Verification items for this drawing (mm, ordinates from the low corner). Give positions to 0.01 mm unless a question says otherwise; leave off trailing zeros. Write each loop counter-clockwise with the first axis right and the second up, starting at its lowest first coordinate (ties: lowest second). Pieces come first, ordered by that corner, then holes. Notation, with made-up numbers: (-20.75, -9) -> (23.25, -9) arc R18 ccw to (23.25, 26) -> close; hole circle Ø4 at (-7, 67.25). An arc over 180 degrees is marked (long way). Write item = value, one per line.
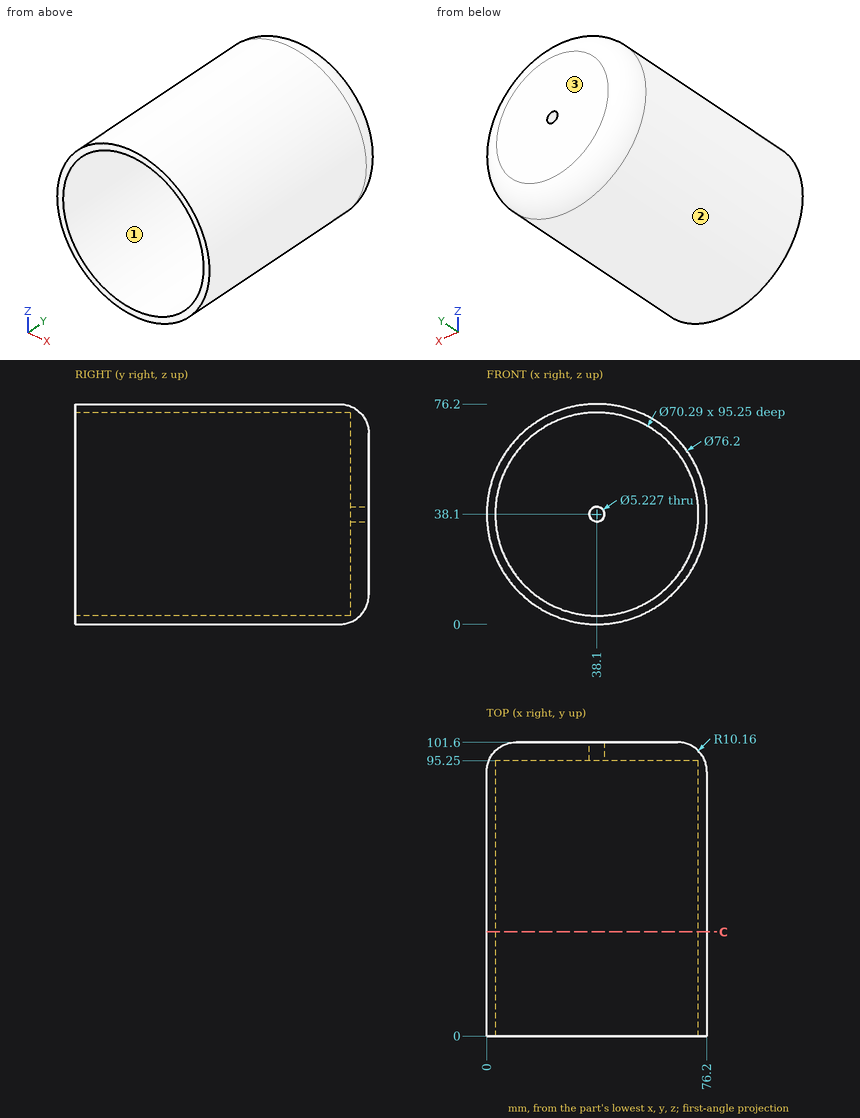
Item 1: Mould release check, pull along Z, two halves, no side actions. Record for the marked faces 1, 2 and 3: +Z half, -Z half, draft (parallel to the pull), parting line (faces both ways), or undercut.
Response values:
face_1 = undercut
face_2 = parting line
face_3 = draft
Item 2: Go/stop test with flat-tipped pins: P1, Ø1.5, axis at x = 64, y = 77, coming from the -Z side; P2, Ø10, axis at y = 51.5, z = 64, coming from the -X side; P3, Ø7, axis at x = 38.1, z = 38.1, coming from the -Y side. Record where each tip stops, or that it passes through.
Response values:
P1 = 9.48
P2 = 6.24
P3 = 95.25
Item 3: Material ranges on line 1 (X direction, y = 51, z = 38) (1 decimal); line 2 (Z direction, x = 24, y = 90.5) (1 decimal), recorded low to high.
Response values:
line_1 = 0 to 3, 73.2 to 76.2
line_2 = 2.7 to 5.9, 70.3 to 73.5
Item 4: Sectioned sample at C-C on y = 36. Record the cut outline in (x, z) (1 decimal).
Response values:
outline = circle Ø76.2 at (38.1, 38.1); hole circle Ø70.3 at (38.1, 38.1)
